```python
from build123d import *

# Parameters (mm, degrees)
SKETCH1_R           = 4.5
BOSS_EXTRUDE1_DEPTH = 8
SKETCH2_R           = 3.5
CUT_EXTRUDE1_DEPTH  = 6.5
BOSS_EXTRUDE2_DEPTH = 2.5


with BuildPart() as part:
    # Sketch1 → Boss-Extrude1 (new body)
    with BuildSketch(Plane.XY):
        Circle(SKETCH1_R)
    extrude(amount=BOSS_EXTRUDE1_DEPTH)

    # Sketch2 → Cut-Extrude1 (cut)
    with BuildSketch(Plane.XY.offset(8)):
        Circle(SKETCH2_R)
    extrude(amount=-CUT_EXTRUDE1_DEPTH, mode=Mode.SUBTRACT)

    # Sketch3 → Boss-Extrude2 (add)
    with BuildSketch(Plane.XY.offset(8)):
        with BuildLine():
            Line((0, 5.25), (0, 3.5))
            ThreePointArc((0, 3.5), (-1.339392013, 3.233578364), (-2.474873734, 2.474873734))
            Line((-2.474873734, 2.474873734), (-3.712310601, 3.712310601))
            ThreePointArc((-3.712310601, 3.712310601), (-2.00908802, 4.850367546), (0, 5.25))
        make_face()
        with BuildLine():
            Line((-5.25, 0), (-3.5, 0))
            ThreePointArc((-3.5, 0), (-3.233578364, -1.339392013), (-2.474873734, -2.474873734))
            Line((-2.474873734, -2.474873734), (-3.712310601, -3.712310601))
            ThreePointArc((-3.712310601, -3.712310601), (-4.850367546, -2.00908802), (-5.25, 0))
        make_face()
        with BuildLine():
            Line((2.474873734, 2.474873734), (3.712310601, 3.712310601))
            ThreePointArc((3.712310601, 3.712310601), (4.850367546, 2.00908802), (5.25, 0))
            Line((5.25, 0), (3.5, 0))
            ThreePointArc((3.5, 0), (3.233578364, 1.339392013), (2.474873734, 2.474873734))
        make_face()
        with BuildLine():
            Line((0, -3.5), (0, -5.25))
            ThreePointArc((0, -5.25), (2.00908802, -4.850367546), (3.712310601, -3.712310601))
            Line((3.712310601, -3.712310601), (2.474873734, -2.474873734))
            ThreePointArc((2.474873734, -2.474873734), (1.339392013, -3.233578364), (0, -3.5))
        make_face()
    extrude(amount=BOSS_EXTRUDE2_DEPTH)


solid = part.part
```
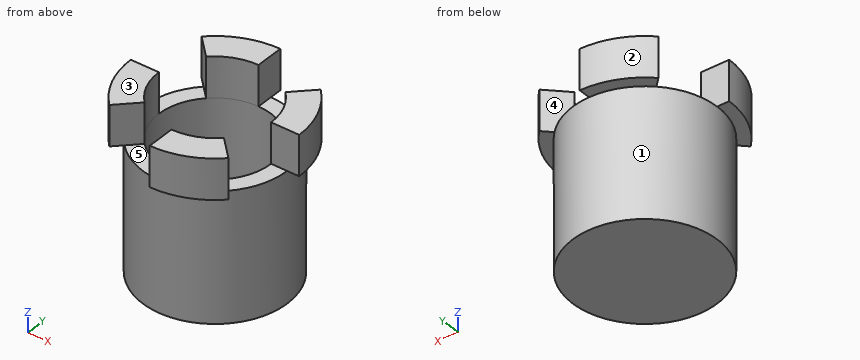
For this review, take the finished solid that the model builds, in its own axes (mm). Face numbers are marked on the shaded views. A direction names the side the tool comes from. Coordinates: 2 decimals unless noted, no trailing zeros. Loops run counter-clockwise (first coordinate to the right, second up) from the corner with the lowest first, then second, coordinate; pieces in that order, holes last.
1. Add section C-C, the plane z = 3. Give the boundary of the cut face in (x, y).
2. For the marked faces 1, 2, 3, 4 and 5, list the 3-axis set-ups (+Z, -Z, +X, -X, +Y, -Y) from which the entire face can be reached by the end or side of a thin tool; tool diameter is ignored.
3. Add section B-B, the plane x = -1.5. Give the boundary of the cut face in (y, z), then the cut area to 3 significant figures.
4. Add section A-A, the plane y = -1. Give the boundary of the cut face in (x, z), then the cut area to 3 significant figures.
5. Add section D-D, the plane y = 3. Give the boundary of the cut face in (x, z), then the cut area to 3 significant figures.
6. Insertion check: P1, Ø5, axis at x = 1.5, z = 4, coming from the -Y side; P2, Ø1, axis at x = -3, y = 1, coming from the +Z side; P3, Ø1, axis at x = 1.5, y = 2.5, coming from the +Z side. Each pin has a flat end and moves straight along its axis. Give the tip position at first contact, or say it passes through.
7. For line 1 (X direction, y = 0, z = 3.25); line 2 (Y direction, x = 1, z = 5.5), list the stretches that pass through material, from the lowest coordinate up.
Result:
1. outline: circle Ø9 at (0, 0); hole circle Ø7 at (0, 0)
2. face 1: -Z
2. face 2: +Z, -Z, -X, +Y
2. face 3: +Z, +X, -X, +Y, -Y
2. face 4: +Z, +Y
2. face 5: +Z, -Y
3. outline: (-4.24, 0) - (4.24, 0) - (4.24, 8) - (5.03, 8) - (5.03, 10.5) - (3.16, 10.5) - (3.16, 1.5) - (-3.16, 1.5) - (-3.16, 8) - (-4.24, 8) - close
3. area: 31.4 mm2
4. outline: (-5.15, 8) - (-4.39, 8) - (-4.39, 0) - (4.39, 0) - (4.39, 8) - (3.35, 8) - (3.35, 1.5) - (-3.35, 1.5) - (-3.35, 10.5) - (-5.15, 10.5) - close
4. area: 31.1 mm2
5. outline: (-3.35, 0) - (3.35, 0) - (3.35, 8) - (4.31, 8) - (4.31, 10.5) - (3, 10.5) - (3, 8) - (1.8, 8) - (1.8, 1.5) - (-1.8, 1.5) - (-1.8, 10.5) - (-3, 10.5) - (-3, 8) - (-3.35, 8) - close
5. area: 36.5 mm2
6. P1: stops at y = -4.5
6. P2: stops at z = 8
6. P3: stops at z = 1.5
7. line 1: x = -4.5 to -3.5, 3.5 to 4.5
7. line 2: y = -4.39 to -3.35, 3.35 to 4.39
